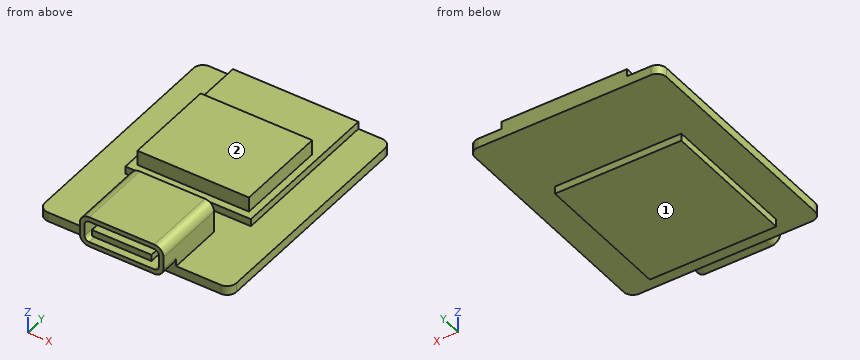
Autodesk Inventor part; units mm, degrees
ref_plane "YZ Plane" through (0, 0, 0) normal (1, 0, 0) x (0, 1, 0)
ref_plane "XZ Plane" through (0, 0, 0) normal (0, 1, 0) x (-1, 0, 0)
ref_plane "XY Plane" through (0, 0, 0) normal (0, 0, 1) x (1, 0, 0)
sketch "Skizze1" plane through (0, 0, 0) normal (0, 0, 1) x (1, 0, 0)
  line L0 (-9.3, 12.75) -> (9.3, 12.75)
  line L1 (10.3, 11.75) -> (10.3, -11.75)
  line L2 (9.3, -12.75) -> (-9.3, -12.75)
  line L3 (-10.3, -11.75) -> (-10.3, 11.75)
  line L4 (-10.3, 12.75) -> (10.3, -12.75) construction
  line L5 (10.3, 12.75) -> (-10.3, -12.75) construction
  arc A0 (-9.3, 12.75) -> (-10.3, 11.75) centre (-9.3, 11.75) ccw
  arc A1 (10.3, 11.75) -> (9.3, 12.75) centre (9.3, 11.75) ccw
  arc A2 (9.3, -12.75) -> (10.3, -11.75) centre (9.3, -11.75) ccw
  arc A3 (-10.3, -11.75) -> (-9.3, -12.75) centre (-9.3, -11.75) ccw
  point P0 (0, 0)
  dimension "d0" = 20.6
  dimension "d1" = 25.5
  dimension "d2" = 1
extrude "Extrusion1" add sketch "Skizze1" along normal blind 1
sketch "Skizze2" plane through (0, 0, 1) normal (0, 0, 1) x (1, 0, 0)
  line L0 (9.3, 12.75) -> (-9.3, 12.75)
  line L1 (-6.75, 12.75) -> (6.75, 12.75)
  line L2 (6.75, 12.75) -> (6.75, -4.25)
  line L3 (6.75, -4.25) -> (-6.75, -4.25)
  line L4 (-6.75, -4.25) -> (-6.75, 12.75)
  line L5 (-10.3, 11.75) -> (-10.3, -11.75)
  line L6 (10.3, -11.75) -> (10.3, 11.75)
  point P0 (0, 0)
  point P1 (6.75, 12.75)
  dimension "d5" = 13.5
  dimension "d6" = 3.55
  dimension "d7" = 3.55
  dimension "d8" = 17
extrude "Extrusion2" add sketch "Skizze2" along normal blind 0.8
sketch "Skizze3" plane through (0, 0, 1.8) normal (0, 0, 1) x (1, 0, 0)
  line L0 (6, -3.45) -> (-6, -3.45)
  line L1 (-6, -3.45) -> (-6, 6.55)
  line L2 (-6, 6.55) -> (6, 6.55)
  line L3 (6, 6.55) -> (6, -3.45)
  line L4 (-6.75, -4.25) -> (6.75, -4.25)
  point P0 (0, 0)
  dimension "d11" = 10
  dimension "d12" = 12
  dimension "d13" = 6
  dimension "d14" = 0.8
extrude "Extrusion3" add sketch "Skizze3" along normal blind 1.6
sketch "Skizze4" plane through (0, 0, 1) normal (0, 0, 1) x (1, 0, 0)
  line L0 (4.5, -14.75) -> (-4.5, -14.75)
  line L1 (-4.5, -14.75) -> (-4.5, -6.75)
  line L2 (-4.5, -6.75) -> (4.5, -6.75)
  line L3 (4.5, -6.75) -> (4.5, -14.75)
  line L4 (-9.3, -12.75) -> (9.3, -12.75)
  point P0 (0, 0)
  dimension "d17" = 9
  dimension "d18" = 4.5
  dimension "d19" = 2
  dimension "d20" = 8
extrude "Extrusion4" add sketch "Skizze4" along normal blind 3.3
fillet "Rundung1" radius 1 4 edges at (-4.5, -10.75, 4.3) (4.5, -10.75, 4.3) (-4.5, -13.75, 1) (4.5, -13.75, 1)
sketch "Skizze5" plane through (-3.5, -14.75, 1) normal (0, -1, 0) x (1, 0, 0)
  arc A0 (7, 0) -> (8, 1) centre (7, 1) ccw
  line L0 (8, 1) -> (8, 2.3)
  arc A1 (8, 2.3) -> (7, 3.3) centre (7, 2.3) ccw
  line L1 (0, 3.3) -> (7, 3.3)
  arc A2 (0, 3.3) -> (-1, 2.3) centre (0, 2.3) ccw
  line L2 (-1, 1) -> (-1, 2.3)
  arc A3 (-1, 1) -> (0, 0) centre (0, 1) ccw
  line L3 (0, 0) -> (7, 0)
  arc A4 (7.5, 2.3) -> (7, 2.8) centre (7, 2.3) ccw
  line L4 (7.5, 2.3) -> (7.5, 1)
  arc A5 (7, 0.5) -> (7.5, 1) centre (7, 1) ccw
  line L5 (7, 0.5) -> (0, 0.5)
  arc A6 (-0.5, 1) -> (0, 0.5) centre (0, 1) ccw
  line L6 (-0.5, 1) -> (-0.5, 2.3)
  arc A7 (0, 2.8) -> (-0.5, 2.3) centre (0, 2.3) ccw
  line L7 (0, 2.8) -> (7, 2.8)
  line L8 (6.7, 2) -> (6.7, 1.3)
  line L9 (6.7, 1.3) -> (0.3, 1.3)
  line L10 (0.3, 1.3) -> (0.3, 2)
  line L11 (0.3, 2) -> (6.7, 2)
  point P0 (3.5, -1)
  dimension "d24" = 0.5
  dimension "d25" = 0.8
extrude "Extrusion5" cut sketch "Skizze5" against normal blind 3.3 contours L4 A5 L5 A6 L6 A7 L7 A4
sketch "Skizze6" plane through (0, 0, 0) normal (0, 0, -1) x (-1, 0, 0)
  line L0 (-6.8, 4.25) -> (6.8, 4.25)
  line L1 (6.8, 4.25) -> (6.8, -10.75)
  line L2 (6.8, -10.75) -> (-6.8, -10.75)
  line L3 (-6.8, -10.75) -> (-6.8, 4.25)
  line L4 (10.3, 11.75) -> (10.3, -11.75)
  line L5 (-10.3, -11.75) -> (-10.3, 11.75)
  line L6 (-9.3, 12.75) -> (9.3, 12.75)
  line L7 (9.3, -12.75) -> (-9.3, -12.75)
  point P0 (0, 0)
  dimension "d28" = 3.5
  dimension "d29" = 3.5
  dimension "d30" = 8.5
  dimension "d31" = 2
extrude "Extrusion6" add sketch "Skizze6" along normal blind 0.8
equation "\"d6\" = d7"
equation "\"d29\" = d28"
properties part number "C3"
Design review of the part built by this model. Coordinates are the model's own, in mm. Face numbers are marked on the shaded views. A direction names the side the tool comes from. Coordinates: 2 decimals unless noted, no trailing zeros. Loops run counter-clockwise (first coordinate to the right, second up) from the corner with the lowest first, then second, coordinate; pieces in that order, holes last. Notation, with made-up numbers: (61.25, -23) - (87.25, -23) arc R25 ccw to (87.25, 13) - close; hole circle Ø1 at (14.25, 70.5). An arc over 180 degrees is marked (long way). Use CSV: the item, a comma, the result in double quotes. Start each with the question number.
1. Add section A-A on z = 2.6. Give the boundary of the cut face in (x, y), plus the area to 3 significant figures.
2. Add section D-D on z = 0.45. Give the boundary of the cut face in (x, y), plus the area to 3 significant figures.
3. Add section B-B on x = -2.5. Give the boundary of the cut face in (y, z).
4. Clearance check with flat-ended pins moving along their axes: pin 1 (0.9 mm diameter, centred on x = -3.5, z = -0.5, fed in from -Y); pin 2 (1.7 mm diameter, centred on x = 1, y = -13.5, fed in from -Z); pin 3 (0.6 mm diameter, centred on y = -13, z = 2.5, fed in from +X). State where each tip first meets the part, or that it passes through.
5. To check wall thickness, follow probe 1 along X at (y, z) = (-13.5, 2.65); probe 2 along Y at (x, z) = (4.25, 1.3); probe 3 along Y at (x, z) = (-0.5, 1.95). State the ranges of each line that lie inside material, in increasing order.
6. For the marked faces 1 and 2, list the 3-axis set-ups (+Z, -Z, +X, -X, +Y, -Y) from which the entire face can be reached by the end or side of a thin tool; tool diameter is ignored.
7. Add section C-C on y = 11.25. Give the boundary of the cut face in (x, z), plus the area to 3 significant figures.
Resolved:
1,outline,"(-6, -3.45) - (6, -3.45) - (6, 6.55) - (-6, 6.55) - close; (-4.5, -14.75) - (-4, -14.75) - (-4, -11.45) - (-3.2, -11.45) - (-3.2, -14.75) - (3.2, -14.75) - (3.2, -11.45) - (4, -11.45) - (4, -14.75) - (4.5, -14.75) - (4.5, -6.75) - (-4.5, -6.75) - close"
1,area,"187 mm2"
2,outline,"(-10.3, -11.75) arc R1 ccw to (-9.3, -12.75) - (9.3, -12.75) arc R1 ccw to (10.3, -11.75) - (10.3, 11.75) arc R1 ccw to (9.3, 12.75) - (-9.3, 12.75) arc R1 ccw to (-10.3, 11.75) - close"
2,area,"524 mm2"
3,outline,"(-14.75, 1) - (-12.75, 1) - (-12.75, 0) - (-10.75, 0) - (-10.75, -0.8) - (4.25, -0.8) - (4.25, 0) - (12.75, 0) - (12.75, 1.8) - (6.55, 1.8) - (6.55, 3.4) - (-3.45, 3.4) - (-3.45, 1.8) - (-4.25, 1.8) - (-4.25, 1) - (-6.75, 1) - (-6.75, 4.3) - (-14.75, 4.3) - (-14.75, 3.8) - (-11.45, 3.8) - (-11.45, 3) - (-14.75, 3) - (-14.75, 2.3) - (-11.45, 2.3) - (-11.45, 1.5) - (-14.75, 1.5) - close"
4,pin 1,"y = -10.75"
4,pin 2,"z = 0"
4,pin 3,"x = 4.5"
5,probe 1,"-4.5 to -4, -3.2 to 3.2, 4 to 4.5"
5,probe 2,"-12.75 to -6.75, -4.25 to 12.75"
5,probe 3,"-11.45 to -6.75, -3.45 to 6.55"
6,face 1,"-Z, +X, -X, +Y, -Y"
6,face 2,"+Z, +X, -X, +Y"
7,outline,"(-10.3, 0) - (10.3, 0) - (10.3, 1) - (6.75, 1) - (6.75, 1.8) - (-6.75, 1.8) - (-6.75, 1) - (-10.3, 1) - close"
7,area,"31.4 mm2"
